Could you check a few things on this drawing? It's one solid part, dimensions in mm from its lowest x, y, z. A direction names the side the tool comes from. Give positions to 0.01 mm unless a question says otherwise; leave off trailing zeros. Write each loop counter-clockwise with the first axis right and the second up, starting at its lowest first coordinate (ties: lowest second). Pieces come first, ordered by that corner, then holes. Notation, with made-up numbers: (62, 24.25) -> (85, 24.25) arc R21 ccw to (85, 51.25) -> close; hole circle Ø7 at (12.5, -36.5). An arc over 180 degrees is marked (long way). Use CSV: the item, a comma, the result in double quotes. Start each with the question number.
(1) I need wall thicknesses on L1, parallel to Z at x = 20, y = 6.5; L2, parallel to Z at x = 119.5, y = 7.5; L3, parallel to Z at x = 23, y = 2. Which ranges of each line are inside material? Lowest first, please. Write a range as [from, to].
(2) Which directions (+Z, -Z, +X, -X, +Y, -Y) give clear straight access to the entire face, cutting with the end or side of a thin tool? Please do the marked faces 5 and 6.
(3) Suppose I cut it at A-A on x = 137.5. List the corners of the cut face in (y, z) for me, plus the area to 3 significant figures.
(4) Suppose I cut it at C-C on y = 6. List the corners of the cut face in (x, z) for me, plus the area to 3 significant figures.
(5) Suppose I cut it at B-B on x = 40. List the corners of the cut face in (y, z) for me, plus the area to 3 significant figures.
(6) If we mould it in two halves opening along Z, with no side actions, what happens to the marked faces 1, 2, 3 and 4? For each: pulls with the +Z half, pulls with the -Z half, needs draft (parallel to the pull), parting line crosses it, or undercut.
(7) For pin 1 Ø1.5 at (y, z) = (3.5, 43.5) entering from +X, with a flat end and sliding along its axis, tell me the tip position at first contact or that it passes through.
(8) Suppose I cut it at D-D on z = 23. List the corners of the cut face in (x, y) for me.
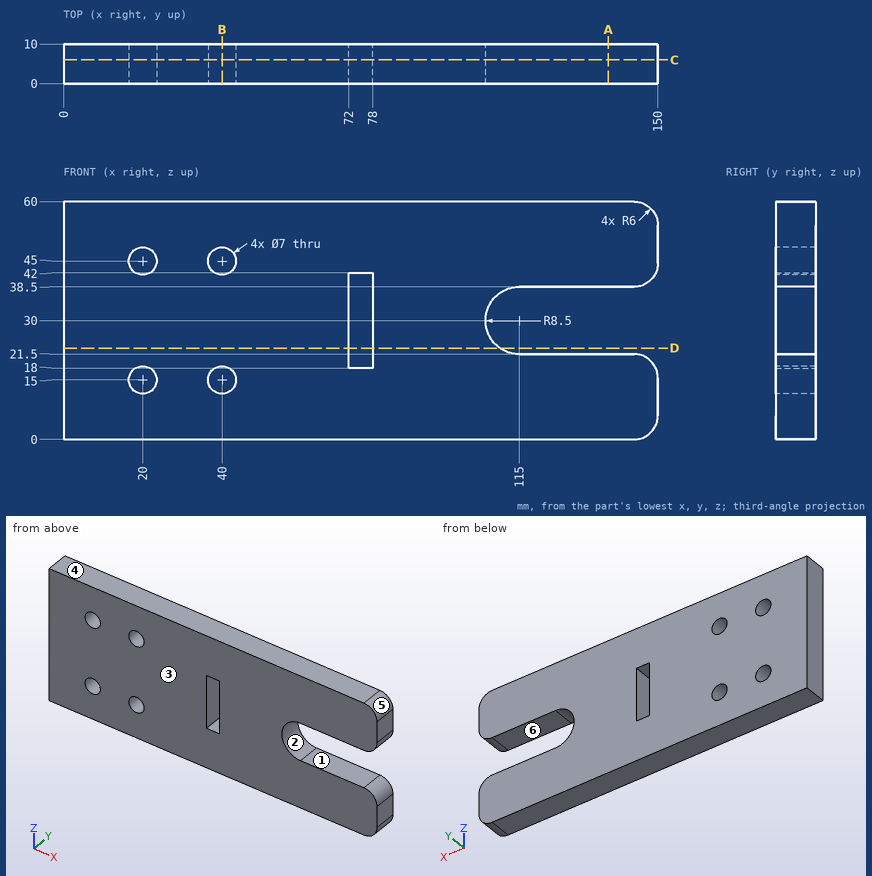
Geometry says:
1,L1,"[0, 11.5], [18.5, 41.5], [48.5, 60]"
1,L2,"[0, 21.5], [38.5, 60]"
1,L3,"[0, 13.2], [16.8, 43.2], [46.8, 60]"
2,face 5,"+Z, +X, +Y, -Y"
2,face 6,"+X, +Y, -Y"
3,outline,"(0, 0) -> (10, 0) -> (10, 21.5) -> (0, 21.5) -> close; (0, 38.5) -> (10, 38.5) -> (10, 60) -> (0, 60) -> close"
3,area,"430 mm²"
4,outline,"(0, 0) -> (144, 0) arc R6 ccw to (150, 6) -> (150, 15.5) arc R6 ccw to (144, 21.5) -> (115, 21.5) arc R8.5 cw to (115, 38.5) -> (144, 38.5) arc R6 ccw to (150, 44.5) -> (150, 54) arc R6 ccw to (144, 60) -> (0, 60) -> close; hole circle Ø7 at (20, 15); hole circle Ø7 at (20, 45); hole circle Ø7 at (40, 15); hole circle Ø7 at (40, 45); hole (72, 18) -> (78, 18) -> (78, 42) -> (72, 42) -> close"
4,area,"7,960 mm²"
5,outline,"(0, 0) -> (10, 0) -> (10, 11.5) -> (0, 11.5) -> close; (0, 18.5) -> (10, 18.5) -> (10, 41.5) -> (0, 41.5) -> close; (0, 48.5) -> (10, 48.5) -> (10, 60) -> (0, 60) -> close"
5,area,"460 mm²"
6,face 1,"undercut"
6,face 2,"undercut"
6,face 3,"needs draft"
6,face 4,"pulls with the +Z half"
7,pin 1,"x = 149.99"
8,outline,"(0, 0) -> (72, 0) -> (72, 10) -> (0, 10) -> close; (78, 0) -> (110.18, 0) -> (110.18, 10) -> (78, 10) -> close"
